```python
from build123d import *

# Parameters (mm, degrees)
BOSS_EXTRUDE2_START = 4
BOSS_EXTRUDE2_DEPTH = 3


with BuildPart() as part:
    # Sketch1 → Revolve1 (revolve)
    with BuildSketch(Plane.XY, mode=Mode.PRIVATE) as revolve1_sk:
        with BuildLine():
            Line((9.5, 0), (11, 0))
            Line((11, 0), (11, 0.6))
            Line((11, 0.6), (8.75, 2))
            ThreePointArc((8.75, 2), (4.447541456, 3.196711086), (0, 3.6))
            Line((0, 3.6), (0, -11.4))
            Line((0, -11.4), (9.5, -11.4))
            Line((9.5, -11.4), (9.5, 0))
        make_face()
    revolve(revolve1_sk.sketch.rotate(Axis((0, 3.6, 0), (0, 1, 0)), 90), axis=Axis((0, 3.6, 0), (0, 1, 0)))

    # Sketch3 → Boss-Extrude2 (add)
    with BuildSketch(Plane.XZ.offset(BOSS_EXTRUDE2_START)):
        Polygon((0, 12.701705922), (-11, 6.350852961), (-11, -6.350852961), (0, -12.701705922), (11, -6.350852961), (11, 6.350852961), align=None)
    extrude(amount=BOSS_EXTRUDE2_DEPTH)


solid = part.part
```
Could you check a few things on this model? Use its own coordinates, in mm. A direction names the side the tool comes from. Round coordinates to 2 decimals unless told otherwise and drop trailing zeros. Write each loop counter-clockwise with the first axis right and the second up, starting at its lowest first coordinate (ties: lowest second). Pieces come first, ordered by that corner, then holes.
(1) Suppose I cut it at C-C on y = -1.5. Write out the boundary of the cut face in (x, z), and give its area (3 significant figures).
Findings below:
outline: circle Ø19 at (0, 0)
area: 284 mm2
(2) Which directions (+Z, -Z, +X, -X, +Y, -Y) give clear straight access to the entire face, cutting with the end or side of a thin tool? Please do faces 1 (the face through (9.274, -1.972, 2.059)), 2 (the face through (10.74, 0.3, 2.38)), 3 (the face through (9.274, -9.169, 2.059)).
Findings below:
face 1: none
face 2: +Y
face 3: -Y
(3) For pin 1 (4 mm diameter, centred on x = -6, z = -3, fed in from +Y); pin 2 (6.5 mm diameter, centred on x = 2, z = 3.5, fed in from +Y); pin 3 (1.5 mm diameter, centred on x = 6, z = -10, fed in from +Y), each with a flat end and sliding along its axis, tell me the tip position at first contact or that it passes through.
Findings below:
pin 1: stops at y = 3.15
pin 2: stops at y = 3.59
pin 3: stops at y = 0.65
(4) Suppose I cut it at D-D on y = 1.25. Write out the boundary of the cut face in (x, z), and give its area (3 significant figures).
Findings below:
outline: circle Ø19.91 at (0, 0)
area: 311 mm2
(5) If I drill on probe 1 along Y at (x, z) = (4.25, 9.5); probe 2 along Y at (x, z) = (0, 7); probe 3 along Y at (x, z) = (-7.75, -2), over which ranges is the centre line in solid material (lowest first)?
Findings below:
probe 1: y = -7 to -4, 0 to 0.97
probe 2: y = -11.4 to 2.59
probe 3: y = -11.4 to 2.27
(6) Suppose I cut it at A-A on z = 0. Write out the boundary of the cut face in (x, y), and give its area (3 significant figures).
Findings below:
outline: (-11, -7) - (-9.5, -7) - (-9.5, -11.4) - (9.5, -11.4) - (9.5, -7) - (11, -7) - (11, -4) - (9.5, -4) - (9.5, 0) - (11, 0) - (11, 0.6) - (8.75, 2) arc R24.73 ccw to (-8.75, 2) - (-11, 0.6) - (-11, 0) - (-9.5, 0) - (-9.5, -4) - (-11, -4) - close
area: 285 mm2
(7) Thinking about a two-plate mould opening in Y: for faces 4 (the face through (4.8, -7, -8.4)), 5 (the face through (4.8, -4, -8.4)), 6 (the face through (5.58, -5.48, 9.48)), which applies, +Y half, -Y half, draft (parallel to the pull), parting line (faces both ways), or undercut?
Findings below:
face 4: -Y half
face 5: undercut
face 6: draft
(8) Suppose I cut it at B-B on y = -5.25. Write out the boundary of the cut face in (x, z).
Findings below:
outline: (-11, -6.35) - (0, -12.7) - (11, -6.35) - (11, 6.35) - (0, 12.7) - (-11, 6.35) - close
